Build history of the part. All positions in model axes, mm. A direction names the side the tool comes from. Coordinates: 2 decimals unless noted, no trailing zeros. Loops run counter-clockwise (first coordinate to the right, second up) from the corner with the lowest first, then second, coordinate; pieces in that order, holes last.
Item 1: Flat gauge pins, fed straight in: pin 1 (3 mm diameter, centred on x = 0, y = 5.5, fed in from +Z); pin 2 (4.5 mm diameter, centred on x = 1, y = 22, fed in from -Z); pin 3 (1.6 mm diameter, centred on x = 0, z = 1, fed in from +Y). Where does each tip first touch, or does it go through?
Item 2: 3-axis set-ups, long thin cutter, end or side, ignore diameter. For faces 5 (the face through (0, 5, 3.15)), 6 (the face through (-2.715, 4.64, -1.597)), 7 (the face through (2.715, 4.64, 1.597)), 8 (the face through (0, 19, 0)): which of +Z, -Z, +X, -X, +Y, -Y reach the whole face in a straight line?
Item 3: Cut at A-A (y = 20). List the corners of the cut face in (x, z) (3 decimals).
Item 4: Cut at B-B (y = 2.25). List the corners of the cut face in (x, z), and give its area (3 significant figures).
Item 5: Drill centre lines: line 1 along Z through (x, y) = (-1.75, 2.75); line 2 along X through (y, z) = (6.25, 2.5); line 3 along X through (y, z) = (19.5, -4.25). Where is each one in solid material? Low to high.
Item 6: Mould opens along Z. For faces 1 (the face through (-2.741, 4.64, 1.553)), 2 (the face through (2.741, 4.64, -1.553)), 3 (the face through (0, 22, -2.75)), 4 (the face through (0, 22, 2.75)) say: released by +Z, released by -Z, zero draft, split by the parting line, or undercut.
Item 7: Cut at D-D (y = 11). List the corners of the cut face in (x, z).
Item 8: Cut at C-C (y = 16.5). List the corners of the cut face in (x, z), and give its area (3 significant figures).
from build123d import *

# Parameters (mm, degrees)
BOSS_EXTRU_1_DEPTH      = 15
ESQUISSE4_W             = 5.5
ESQUISSE4_H             = 5.5
ENL_V_MAT_EXTRU_1_DEPTH = 6
CONG_2_R                = 40


with BuildPart() as part:
    # Esquisse1 → Boss.-Extru.1 (new body)
    with BuildSketch(Plane(origin=(0, 0, 0), x_dir=(1, 0, 0), z_dir=(0, 1, 0))):
        Polygon((1.818653348, -3.15), (3.637306696, 0), (1.818653348, 3.15), (-1.818653348, 3.15), (-3.637306696, 0), (-1.818653348, -3.15), align=None)
    extrude(amount=BOSS_EXTRU_1_DEPTH)

    # Esquisse3 → section 1 of lissage1
    with BuildSketch(Plane(origin=(0, 25, 0), x_dir=(1, 0, 0), z_dir=(0, 1, 0)), mode=Mode.PRIVATE) as lissage1_s1:
        with BuildLine():
            Line((3.464101615, -6), (6.92820323, 0))
            Line((6.92820323, 0), (3.464101615, 6))
            Line((3.464101615, 6), (-3.464101615, 6))
            Line((-3.464101615, 6), (-6.92820323, 0))
            Line((-6.92820323, 0), (-3.464101615, -6))
            Line((-3.464101615, -6), (3.464101615, -6))
        make_face()
    # loft from a face of the part (lissage1)
    loft([part.faces().sort_by_distance((0, 15, 0))[0], lissage1_s1.sketch])

    # Esquisse4 → Enlèv. mat.-Extru.1 (cut)
    with BuildSketch(Plane(origin=(0, 25, 0), x_dir=(1, 0, 0), z_dir=(0, 1, 0))):
        Rectangle(ESQUISSE4_W, ESQUISSE4_H)
    extrude(amount=-ENL_V_MAT_EXTRU_1_DEPTH, mode=Mode.SUBTRACT)

    # Congé2
    # the kernel refuses this fillet: 40 mm, written as the material it adds along each edge
    with BuildSketch(Plane(origin=(-15.790476474, 15, 3.15), x_dir=(0, -1, 0), z_dir=(1, 0, 0))) as cong_2_piece_1_section:
        with BuildLine():
            CenterArc((CONG_2_R * 0.139718231259, -CONG_2_R), CONG_2_R, 90, 15.907551931)
            Line((-CONG_2_R * 0.134367748379, -CONG_2_R * 0.0382948082879), (0, 0))
            Line((0, 0), (CONG_2_R * 0.139718231259, 0))
        make_face()
    cong_2_piece_1 = extrude(amount=31.580952948, mode=Mode.PRIVATE)
    cong_2_piece_1 = cong_2_piece_1 - Plane(origin=(-39.952625281, 9.41127075, 17.100023118), x_dir=(0.8660254037844387, 0, -0.5000000000000001), z_dir=(-0.5000000000000001, 0, -0.8660254037844387)) * Cylinder(40, 86, mode=Mode.PRIVATE)
    cong_2_piece_1 = cong_2_piece_1 - Plane(origin=(32.057387044, 9.41127075, 30.774976882), x_dir=(-0.8660254037844385, 0, -0.5000000000000003), z_dir=(-0.5000000000000003, 0, 0.8660254037844385)) * Cylinder(40, 86, mode=Mode.PRIVATE)
    add(cong_2_piece_1)
    with BuildSketch(Plane(origin=(-5.167258215, 15, 15.249953764), x_dir=(0, -1, 0), z_dir=(0.5000000000000003, 0, -0.8660254037844385))) as cong_2_piece_2_section:
        with BuildLine():
            CenterArc((CONG_2_R * 0.139718231259, -CONG_2_R), CONG_2_R, 90, 15.907551931)
            Line((-CONG_2_R * 0.134367748379, -CONG_2_R * 0.0382948082879), (0, 0))
            Line((0, 0), (CONG_2_R * 0.139718231259, 0))
        make_face()
    cong_2_piece_2 = extrude(amount=31.580952948, mode=Mode.PRIVATE)
    cong_2_piece_2 = cong_2_piece_2 - Plane(origin=(42.680605303, 9.41127075, -12.375023118), x_dir=(-0.8660254037844388, 0, 0.4999999999999999), z_dir=(0.4999999999999999, 0, 0.8660254037844388)) * Cylinder(40, 86, mode=Mode.PRIVATE)
    cong_2_piece_2 = cong_2_piece_2 - Plane(origin=(-5.167258215, 9.41127075, 43.15), x_dir=(0, 0, -1), z_dir=(-1, 0, 0)) * Cylinder(40, 86, mode=Mode.PRIVATE)
    add(cong_2_piece_2)
    with BuildSketch(Plane(origin=(10.623218259, 15, 12.099953764), x_dir=(0, -1, 0), z_dir=(-0.49999999999999994, 0, -0.8660254037844388))) as cong_2_piece_3_section:
        with BuildLine():
            CenterArc((CONG_2_R * 0.139718231259, -CONG_2_R), CONG_2_R, 90, 15.907551931)
            Line((-CONG_2_R * 0.134367748379, -CONG_2_R * 0.0382948082879), (0, 0))
            Line((0, 0), (CONG_2_R * 0.139718231259, 0))
        make_face()
    cong_2_piece_3 = extrude(amount=31.580952948, mode=Mode.PRIVATE)
    cong_2_piece_3 = cong_2_piece_3 - Plane(origin=(34.785367066, 9.41127075, 26.049976882), x_dir=(-0.8660254037844385, 0, -0.5000000000000003), z_dir=(-0.5000000000000003, 0, 0.8660254037844385)) * Cylinder(40, 86, mode=Mode.PRIVATE)
    cong_2_piece_3 = cong_2_piece_3 - Plane(origin=(10.623218259, 9.41127075, -43.15), x_dir=(0, 0, 1), z_dir=(1, 0, 0)) * Cylinder(40, 86, mode=Mode.PRIVATE)
    add(cong_2_piece_3)
    with BuildSketch(Plane(origin=(15.790476474, 15, -3.15), x_dir=(0, -1, 0), z_dir=(-1, 0, 0))) as cong_2_piece_4_section:
        with BuildLine():
            CenterArc((CONG_2_R * 0.139718231259, -CONG_2_R), CONG_2_R, 90, 15.907551931)
            Line((-CONG_2_R * 0.134367748379, -CONG_2_R * 0.0382948082879), (0, 0))
            Line((0, 0), (CONG_2_R * 0.139718231259, 0))
        make_face()
    cong_2_piece_4 = extrude(amount=31.580952948, mode=Mode.PRIVATE)
    cong_2_piece_4 = cong_2_piece_4 - Plane(origin=(-32.057387044, 9.41127075, -30.774976882), x_dir=(0.8660254037844385, 0, 0.5000000000000002), z_dir=(0.5000000000000003, 0, -0.8660254037844386)) * Cylinder(40, 86, mode=Mode.PRIVATE)
    cong_2_piece_4 = cong_2_piece_4 - Plane(origin=(39.952625281, 9.41127075, -17.100023118), x_dir=(-0.8660254037844388, 0, 0.4999999999999999), z_dir=(0.4999999999999999, 0, 0.8660254037844388)) * Cylinder(40, 86, mode=Mode.PRIVATE)
    add(cong_2_piece_4)
    with BuildSketch(Plane(origin=(5.167258215, 15, -15.249953764), x_dir=(0, -1, 0), z_dir=(-0.5000000000000003, 0, 0.8660254037844386))) as cong_2_piece_5_section:
        with BuildLine():
            CenterArc((CONG_2_R * 0.139718231259, -CONG_2_R), CONG_2_R, 90, 15.907551931)
            Line((-CONG_2_R * 0.134367748379, -CONG_2_R * 0.0382948082879), (0, 0))
            Line((0, 0), (CONG_2_R * 0.139718231259, 0))
        make_face()
    cong_2_piece_5 = extrude(amount=31.580952948, mode=Mode.PRIVATE)
    cong_2_piece_5 = cong_2_piece_5 - Plane(origin=(-42.680605303, 9.41127075, 12.375023118), x_dir=(0.8660254037844387, 0, -0.5000000000000001), z_dir=(-0.5000000000000001, 0, -0.8660254037844387)) * Cylinder(40, 86, mode=Mode.PRIVATE)
    cong_2_piece_5 = cong_2_piece_5 - Plane(origin=(5.167258215, 9.41127075, -43.15), x_dir=(0, 0, 1), z_dir=(1, 0, 0)) * Cylinder(40, 86, mode=Mode.PRIVATE)
    add(cong_2_piece_5)
    with BuildSketch(Plane(origin=(-10.623218259, 15, -12.099953764), x_dir=(0, -1, 0), z_dir=(0.5000000000000001, 0, 0.8660254037844387))) as cong_2_piece_6_section:
        with BuildLine():
            CenterArc((CONG_2_R * 0.139718231259, -CONG_2_R), CONG_2_R, 90, 15.907551931)
            Line((-CONG_2_R * 0.134367748379, -CONG_2_R * 0.0382948082879), (0, 0))
            Line((0, 0), (CONG_2_R * 0.139718231259, 0))
        make_face()
    cong_2_piece_6 = extrude(amount=31.580952948, mode=Mode.PRIVATE)
    cong_2_piece_6 = cong_2_piece_6 - Plane(origin=(-34.785367066, 9.41127075, -26.049976882), x_dir=(0.8660254037844385, 0, 0.5000000000000002), z_dir=(0.5000000000000003, 0, -0.8660254037844386)) * Cylinder(40, 86, mode=Mode.PRIVATE)
    cong_2_piece_6 = cong_2_piece_6 - Plane(origin=(-10.623218259, 9.41127075, 43.15), x_dir=(0, 0, -1), z_dir=(-1, 0, 0)) * Cylinder(40, 86, mode=Mode.PRIVATE)
    add(cong_2_piece_6)


solid = part.part
Filled sheet:
1. pin 1: stops at z = 3.15
1. pin 2: stops at z = -5.79
1. pin 3: stops at y = 19
2. face 5: +Z, +X, -X, -Y
2. face 6: -Z, -X, -Y
2. face 7: +Z, +X, -Y
2. face 8: +Y
3. outline: (-5.285, 0) - (-2.643, -4.577) - (2.643, -4.577) - (5.285, 0) - (2.643, 4.577) - (-2.643, 4.577) - close; hole (-2.75, -2.75) - (2.75, -2.75) - (2.75, 2.75) - (-2.75, 2.75) - close
4. outline: (-3.64, 0) - (-1.82, -3.15) - (1.82, -3.15) - (3.64, 0) - (1.82, 3.15) - (-1.82, 3.15) - close
4. area: 34.4 mm2
5. line 1: z = -3.15 to 3.15
5. line 2: x = -2.19 to 2.19
5. line 3: x = -2.68 to 2.68
6. face 1: released by +Z
6. face 2: released by -Z
6. face 3: undercut
6. face 4: undercut
7. outline: (-3.67, 0) - (-1.84, -3.18) - (1.84, -3.18) - (3.67, 0) - (1.84, 3.18) - (-1.84, 3.18) - close
8. outline: (-4.37, 0) - (-2.18, -3.78) - (2.18, -3.78) - (4.37, 0) - (2.18, 3.78) - (-2.18, 3.78) - close
8. area: 49.6 mm2
